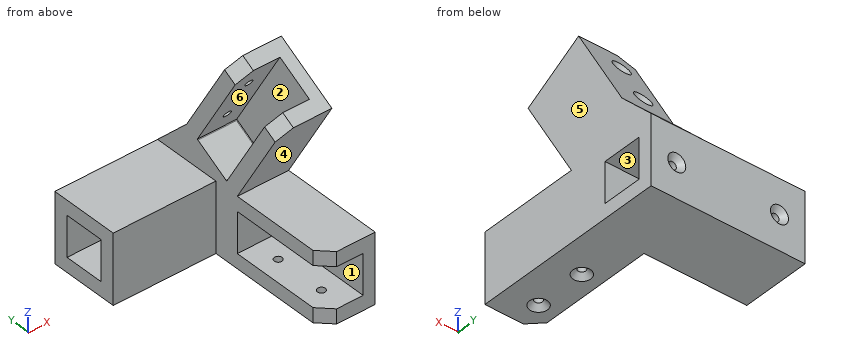
```python
from build123d import *

# Parameters (mm, degrees)
F0_W      = 15
F0_H      = 15
F1_DEPTH  = 20
F2_W      = 40
F2_H      = 15
F3_DEPTH  = 15
F4_W      = 27
F4_H      = 27
F4_W_2    = 15
F4_H_2    = 15
F5_DEPTH  = 60
F6_W      = 15.7
F6_H      = 15.7
F7_DEPTH  = 60.001
F8_W      = 15.7
F8_H      = 15.7
F9_DEPTH  = 40.001
F10_W     = 15.7
F10_H     = 15.7
F11_DEPTH = 61.6923429511
F12_R     = 1.5
F13_DEPTH = 5.65
F14_R     = 1.5
F15_DEPTH = 34.6628510268
F16_R     = 1.5
F17_DEPTH = 5.651
F18_SIZE  = 5
F19_SIZE  = 2
F21_DEPTH = 20


with BuildPart() as f1:
    # F0 (on Right) → F1 (new body)
    with BuildSketch(Plane.YZ):
        Polygon((-63.3826859022, -13.5), (13.5, -13.5), (13.5, 3.6173140978), (-20, 61.6410161514), (-43.3826859022, 48.1410161514), (-23.3826859022, 13.5), (-63.3826859022, 13.5), align=None)
        Rectangle(F0_W, F0_H, mode=Mode.SUBTRACT)
    extrude(amount=-F1_DEPTH)

    # F2 (on face) → F3 (cut)
    with BuildSketch(Plane(origin=(-20, 0, 0), x_dir=(0, -1, 0), z_dir=(-1, 0, 0))):
        Polygon((5.1961524227, 24), (18.1865334795, 16.5), (38.1865334795, 51.1410161514), (25.1961524227, 58.6410161514), align=None)
        with Locations((43.3826859022, 0)):
            Rectangle(F2_W, F2_H)
    extrude(amount=-F3_DEPTH, mode=Mode.SUBTRACT)

    # F4 (on face) → F5 (join)
    with BuildSketch(Plane.YZ):
        Rectangle(F4_W, F4_H)
        Rectangle(F4_W_2, F4_H_2, mode=Mode.SUBTRACT)
    extrude(amount=-F5_DEPTH)

    # F6 (on face) → F7 (cut, through all)
    with BuildSketch(Plane(origin=(-60, 0, 0), x_dir=(0, -1, 0), z_dir=(-1, 0, 0))):
        Rectangle(F6_W, F6_H)
    extrude(amount=-F7_DEPTH, mode=Mode.SUBTRACT)

    # F8 (on face) → F9 (cut, through all)
    with BuildSketch(Plane.XZ.offset(23.3826859022)):
        with Locations((-12.5, 0)):
            Rectangle(F8_W, F8_H)
    extrude(amount=F9_DEPTH, mode=Mode.SUBTRACT)

    # F10 (on face) → F11 (cut, through all)
    with BuildSketch(Plane(origin=(0, -11.6913429511, 20.25), x_dir=(1, 0, 0), z_dir=(0, -0.5, 0.8660254038))):
        with Locations((-12.5, 0)):
            Rectangle(F10_W, F10_H)
    extrude(amount=F11_DEPTH, mode=Mode.SUBTRACT)

    # F12 (on face) → F13 (cut, through all)
    with BuildSketch(Plane(origin=(0, 13.5, 0), x_dir=(-1, 0, 0), z_dir=(0, 1, 0))):
        with Locations((10, 0)):
            Circle(F12_R)
        with Locations((50, 0)):
            Circle(F12_R)
    extrude(amount=-F13_DEPTH, mode=Mode.SUBTRACT)

    # F14 (on face) → F15 (cut, through all)
    with BuildSketch(Plane(origin=(0, 6.7982994197, 3.925), x_dir=(1, 0, 0), z_dir=(0, -0.8660254038, -0.5))):
        with Locations((-12.5, 33.3826859022)):
            Circle(F14_R)
        with Locations((-12.5, 53.3826859022)):
            Circle(F14_R)
    extrude(amount=-F15_DEPTH, mode=Mode.SUBTRACT)

    # F16 (on face) → F17 (cut, through all)
    with BuildSketch(Plane.XY.offset(-7.85)):
        with Locations((-12.5, -53.3826859022)):
            Circle(F16_R)
        with Locations((-12.5, -33.3826859022)):
            Circle(F16_R)
    extrude(amount=-F17_DEPTH, mode=Mode.SUBTRACT)

    # F18
    f18_edges = [f1.edges().sort_by_distance(p)[0] for p in [
        (-20, -40.936164, 49.553516),
        (-20, -22.446522, 60.228516),
        (-20, -63.382686, 10.675),
        (-20, -63.382686, -10.675),
    ]]
    chamfer(f18_edges, length=F18_SIZE)

    # F19
    f19_edges = [f1.edges().sort_by_distance(p)[0] for p in [
        (-14, -15, 52.980762),
        (-14, -5, 35.660254),
        (-8.5, 13.5, 0),
        (-48.5, 13.5, 0),
        (-14, -33.382686, -13.5),
        (-14, -53.382686, -13.5),
    ]]
    chamfer(f19_edges, length=F19_SIZE)

    # F20 (on face) → F21 (join, through all)
    with BuildSketch(Plane.YZ):
        Polygon((7.7942286341, 13.5), (13.5, 13.5), (0, 27), align=None)
    extrude(amount=-F21_DEPTH)


solid = f1.part
```
Part model, mm, in its own coordinate system. Face numbers are marked on the shaded views. A direction names the side the tool comes from. Round coordinates to 2 decimals unless told otherwise and drop trailing zeros. Loops run counter-clockwise (first coordinate to the right, second up) from the corner with the lowest first, then second, coordinate; pieces in that order, holes last. Notation, with made-up numbers: (43, -14.75) -> (97, -14.75) arc R23 ccw to (97, 16.25) -> close; hole circle Ø3 at (-33.5, 76.5). An arc over 180 degrees is marked (long way). Use one line per item in the form item = value. Start each with the question number.
Item 1: Two-plate mould, pull along Y, no slides. Class the marked faces 4, 5 and 6: released by +Y, released by -Y, zero draft, split by the parting line, or undercut.
Item 2: Band-saw the part on D-D (x = -12.5). Give the number of separate pieces and of enclosed holes in the cut face, plus the area to 3 significant figures.
Item 3: Band-saw the part on A-A (x = -33). List the corners of the cut face in (y, z), plus the area to 3 significant figures.
Item 4: Drill centre lines: line 1 along Z through (x, y) = (-40.5, 1); line 2 along Z through (x, y) = (-8, -30.5); line 3 along X through (y, z) = (-23.5, 3). Where is each one in solid material? Low to high.
Item 5: Band-saw the part on C-C (x = -50). List the corners of the cut face in (y, z), plus the area to 3 significant figures.
Item 6: Tool access for the marked faces 1, 2 and 3: list every direction of +Z, -Z, +X, -X, +Y, -Y with a clear straight run to the whole face (end or side of a thin tool).
Item 7: Band-saw the part on B-B (z = 5). List the corners of the cut face in (x, y), plus the area to 3 significant figures.
Item 8: Drop flat-ended pins along their axis: pin 1 Ø6 at (x, y) = (-15, -55) entering from +Z; pin 2 Ø8 at (y, z) = (-29, 44) entering from -X; pin 3 Ø17 at (x, y) = (-12, -43) entering from +Z; pin 4 Ø2 at (x, y) = (-31.5, -15.5) entering from +Z. Give the stop position or say it passes through.
Data:
q1.face_4 = released by -Y
q1.face_5 = zero draft
q1.face_6 = undercut
q2.separate_pieces = 5
q2.enclosed_holes = 1
q2.area = 1,820 mm^2
q3.outline = (-13.5, -13.5) -> (13.5, -13.5) -> (13.5, 13.5) -> (-13.5, 13.5) -> close; hole (-7.85, -7.85) -> (7.85, -7.85) -> (7.85, 7.85) -> (-7.85, 7.85) -> close
q3.area = 483 mm^2
q4.line_1 = -13.5 to -7.85, 7.85 to 13.5
q4.line_2 = -13.5 to -7.85, 7.85 to 13.5, 25.83 to 37.13
q4.line_3 = -4.65 to 0
q5.outline = (-13.5, -13.5) -> (13.5, -13.5) -> (13.5, -3.5) -> (11.5, -1.5) -> (7.85, -1.5) -> (7.85, -7.85) -> (-7.85, -7.85) -> (-7.85, 7.85) -> (7.85, 7.85) -> (7.85, 1.5) -> (11.5, 1.5) -> (13.5, 3.5) -> (13.5, 13.5) -> (-13.5, 13.5) -> close
q5.area = 462 mm^2
q6.face_1 = -X, -Y
q6.face_2 = -X
q6.face_3 = +X, -X
q7.outline = (-60, -13.5) -> (-20, -13.5) -> (-20, -23.38) -> (-4.65, -23.38) -> (-4.65, -63.38) -> (0, -63.38) -> (0, -7.85) -> (-60, -7.85) -> close; (-60, 7.85) -> (0, 7.85) -> (0, 13.5) -> (-60, 13.5) -> close
q7.area = 1,060 mm^2
q8.pin_1 = 13.5
q8.pin_2 = -4.65
q8.pin_3 = 50.97
q8.pin_4 = through
